The drawing under review shows one solid part. Ordinate dimensions are in mm from its lowest x, y, z. A direction names the side the tool comes from. Give positions to 0.01 mm unless a question says otherwise; leave off trailing zeros. Order: outer loops, then holes, each group sorted by start corner. A loop starts at its lowest first (then second) coordinate and runs counter-clockwise, first axis right, second up. Notation, with made-up numbers: (74.5, -8.5) -> (89.5, -8.5) arc R12 cw to (89.5, -1.5) -> close; hole circle Ø6 at (24.5, -27.75). An arc over 180 degrees is marked (long way). One line per item, written item: value. Start each with the question number.
1) Tool access review of the marked faces 4, 5, 6 and 7: name each direction out of +Z, -Z, +X, -X, +Y, -Y from which nothing blocks a thin tool from reaching the whole face with its end or side.
2) For pin 1 (3 mm diameter, centred on x = 9.5, z = 8.5, fed in from +Y); pin 2 (10 mm diameter, centred on x = 3, y = 30, fed in from -Z); pin 3 (1 mm diameter, centred on x = 7.5, z = 5, fed in from -Y); pin 4 (0.5 mm diameter, centred on x = 11.5, y = 33, fed in from +Z), all flat-tipped, find the tip position at first contact; note any pin that passes through.
3) Consider section C-C (z = 16). State the section outline as (x, y) points.
4) The part is to be moulded in two halves that separate along X. For the marked faces 1, 2 and 3, say which applies: released by +X, released by -X, zero draft, split by the parting line, or undercut.
5) Wall thickness on line 1 along Y through (x, z) = (23.25, 9.75); line 2 along Y through (x, z) = (21.5, 4); line 3 along Y through (x, z) = (10, 1.25): over which ranges is each line inside the solid? List them lowest first. Write a range as from..to.
6) Consider section A-A (z = 12). State the section outline as (x, y) points.
7) Consider section B-B (x = 21.5). State the section outline as (y, z) points.
8) Consider section D-D (y = 36). State the section outline as (x, z) points, plus the area to 3 significant figures.
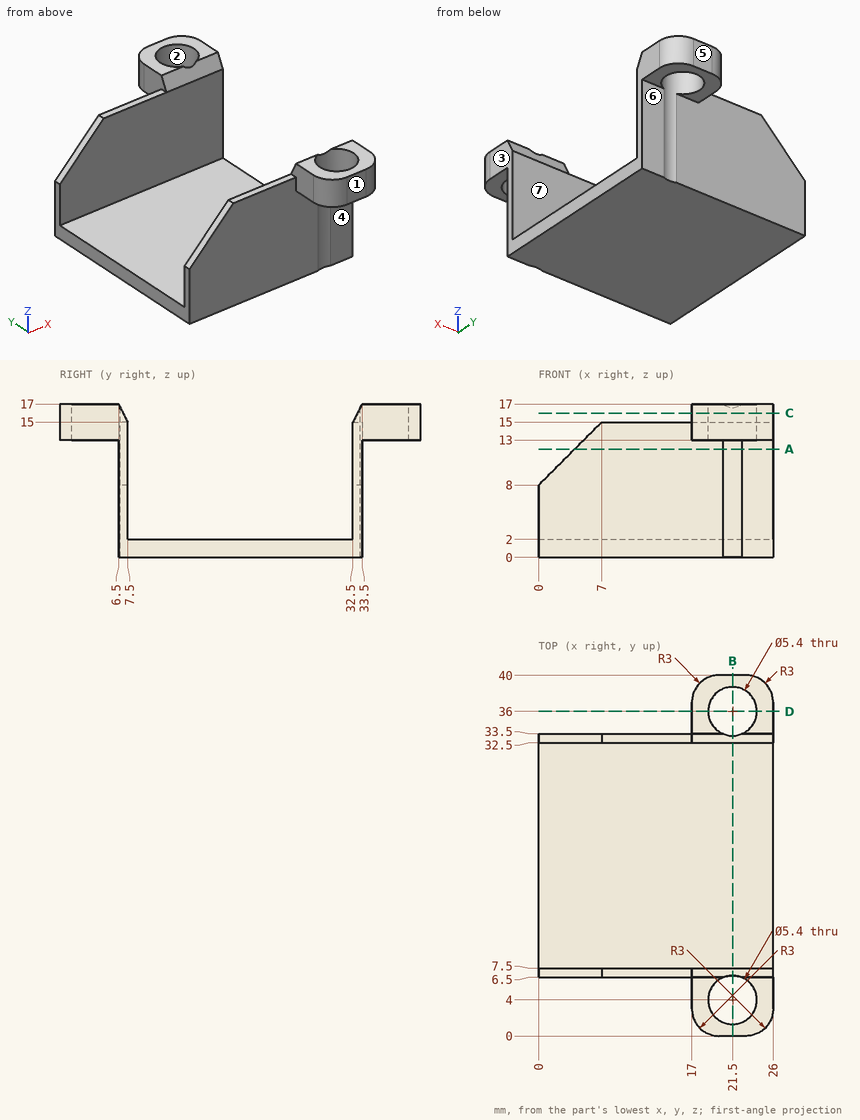
Checked values:
1. face 4: -Z, +X, -X, -Y
1. face 5: +Z, -Z, +X, -X, +Y
1. face 6: -Z, +X, -X, +Y
1. face 7: +Z, +X, -X
2. pin 1: stops at y = 33.5
2. pin 2: stops at z = 0
2. pin 3: stops at y = 6.5
2. pin 4: stops at z = 15
3. outline: (17, 3) arc R3 ccw to (20, 0) -> (23, 0) arc R3 ccw to (26, 3) -> (26, 7) -> (17, 7) -> close; (17, 33) -> (26, 33) -> (26, 37) arc R3 ccw to (23, 40) -> (20, 40) arc R3 ccw to (17, 37) -> close; hole circle Ø5.4 at (21.5, 4); hole circle Ø5.4 at (21.5, 36)
4. face 1: zero draft
4. face 2: undercut
4. face 3: released by +X
5. line 1: y = 6.5..7.5, 32.5..33.5
5. line 2: y = 6.7..7.5, 32.5..33.3
5. line 3: y = 6.5..33.5
6. outline: (4, 6.5) -> (20.48, 6.5) arc R2.7 cw to (22.52, 6.5) -> (26, 6.5) -> (26, 7.5) -> (4, 7.5) -> close; (4, 32.5) -> (26, 32.5) -> (26, 33.5) -> (22.52, 33.5) arc R2.7 cw to (20.48, 33.5) -> (4, 33.5) -> close
7. outline: (0, 13) -> (1.3, 13) -> (1.3, 17) -> (0, 17) -> close; (6.7, 0) -> (33.3, 0) -> (33.3, 16.6) -> (32.5, 15) -> (32.5, 2) -> (7.5, 2) -> (7.5, 15) -> (6.7, 16.6) -> close; (38.7, 13) -> (40, 13) -> (40, 17) -> (38.7, 17) -> close
8. outline: (17, 13) -> (18.8, 13) -> (18.8, 17) -> (17, 17) -> close; (24.2, 13) -> (26, 13) -> (26, 17) -> (24.2, 17) -> close
8. area: 14.4 mm^2
